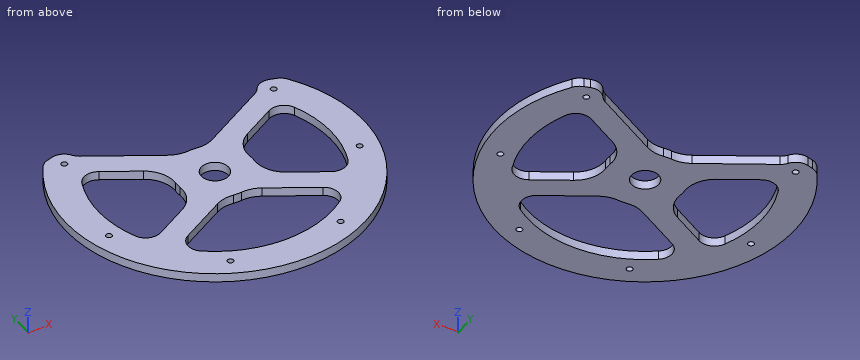
Autodesk Inventor part; units mm, degrees
ref_plane "YZ Plane" through (0, 0, 0) normal (1, 0, 0) x (0, 1, 0)
ref_plane "XZ Plane" through (0, 0, 0) normal (0, 1, 0) x (-1, 0, 0)
ref_plane "XY Plane" through (0, 0, 0) normal (0, 0, 1) x (1, 0, 0)
sketch "スケッチ1" plane through (0, 0, 0) normal (0, 0, 1) x (1, 0, 0)
  circle A0 centre (69, 50) radius 2
  circle A1 centre (0, 0) radius 9
  circle A2 centre (0, 0) radius 25
  circle A3 centre (69, 50) radius 7.5
  line L0 (65.25, 56.4952) -> (8.2643, 23.5945)
  line L1 (0, 25) -> (0, -25)
  line L2 (-25, 0) -> (25, 0)
  line L3 (20.9707, 13.61) -> (72.75, 43.5048)
  circle A4 centre (69, -50) radius 2
  circle A5 centre (69, -50) radius 7.5
  line L4 (65.25, -56.4952) -> (8.2643, -23.5945)
  line L5 (20.9707, -13.61) -> (72.75, -43.5048)
  circle A6 centre (-69, 50) radius 2
  circle A7 centre (-69, 50) radius 7.5
  line L6 (-65.25, 56.4952) -> (-8.2643, 23.5945)
  line L7 (-20.9707, 13.61) -> (-72.75, 43.5048)
  line L8 (-65.25, -56.4952) -> (-8.2643, -23.5945)
  circle A8 centre (-69, -50) radius 7.5
  circle A9 centre (-69, -50) radius 2
  line L9 (-20.9707, -13.61) -> (-72.75, -43.5048)
  circle A10 centre (0, 0) radius 77
  circle A11 centre (0, 0) radius 86.5
  circle A12 centre (0, 0) radius 98.5
  line L10 (0, 0) -> (79.6882, 57.8968)
  line L11 (0, 0) -> (95.4054, -24.496)
  line L12 (0, 0) -> (41.9393, -89.1255)
  line L13 (0, 0) -> (-79.6882, 57.8968)
  line L14 (0, 0) -> (-95.4054, -24.496)
  line L15 (0, 0) -> (-41.9393, -89.1255)
  circle A13 centre (69.98, 50.8434) radius 2
  circle A14 centre (83.7824, -21.5117) radius 2
  circle A15 centre (36.8299, -78.2675) radius 2
  circle A16 centre (69.98, 50.8434) radius 9.5
  circle A17 centre (-69.98, 50.8434) radius 2
  circle A18 centre (-83.7824, -21.5117) radius 2
  circle A19 centre (-36.8299, -78.2675) radius 2
  circle A20 centre (-69.98, 50.8434) radius 9.5
  line L16 (-79.6882, 57.8968) -> (-72.6529, 59.9596)
  line L17 (79.6882, 57.8968) -> (72.6529, 59.9596)
  point P0 (-8.2643, 23.5945)
  point P1 (-8.2643, -23.5945)
  point P2 (8.2643, -23.5945)
  point P3 (66.0238, -39.6214)
  point P4 (57.0218, -51.7447)
  point P5 (-57.0218, -51.7447)
  point P6 (-66.0238, -39.6214)
  point P7 (-66.0238, 39.6214)
  point P8 (-57.0218, 51.7447)
  point P9 (-62.2943, 45.2595)
  point P10 (-77.6656, 56.4274)
  point P11 (77.6656, 56.4274)
  point P12 (62.2943, 45.2595)
  point P13 (57.0218, 51.7447)
  point P14 (66.0238, 39.6214)
  point P15 (-61.0434, 54.0665)
  point P16 (61.0434, 54.0665)
  point P17 (69.0803, 41.3861)
  point P18 (-69.0803, 41.3861)
  point P19 (-12.1615, -25.8445)
  point P20 (-10.6445, -22.6207)
  point P21 (10.6445, -22.6207)
  point P22 (12.1615, -25.8445)
  dimension "d19" = 19
  dimension "d0" = 4
  dimension "d1" = 50
  dimension "d2" = 69
  dimension "d3" = 18
  dimension "d4" = 50
  dimension "d5" = 15
  dimension "d6" = 30
  dimension "d10" = 154
  dimension "d11" = 173
  dimension "d12" = 197
  dimension "d13" = 54
  dimension "d14" = 50.4
  dimension "d15" = 50.4
  dimension "d16" = 4
  dimension "d17" = 4
  dimension "d18" = 4
extrude "押し出し1" add sketch "スケッチ1" along normal blind 5.8 contours A13 A11 A3 L10 | L10 A3 A11 A13 | A13 A11 A3 L10 A0 | A0 L10 A13 | A13 L10 A0 | A0 L10 A3 A11 A13 | L10 A16 A11 A3 | A3 A11 A16 L10 | A11 A16 L3 A3 | A3 L0 A16 A11 | A16 L17 L10 | L10 A12 L11 A14 A11 A16 | L10 A16 L0 A3 | A3 L3 A16 L10 | A11 A14 L11 A10 L3 A16 | A16 L3 A10 | L10 A2 L0 A10 | A10 L3 A2 L10 | A10 L0 A16 | A20 L6 A7 A11 | A11 A7 L13 A20 | L13 A20 A11 A18 L14 A12 | L16 A20 L13 | L10 A1 L1 A2 | A2 L2 A1 L10 | A11 A17 L13 A7 | A7 L13 A6 A17 A11 | A20 L13 A7 L6 | L6 A10 A20 | A12 L12 A15 A11 A5 A14 L11 | L14 A18 A11 A8 A19 L15 A12 | L13 A7 A11 A20 | L6 A2 L13 A10 | A14 A11 A5 L5 A10 L11 | L13 A17 A11 A7 | A12 L15 A19 A11 A15 L12 | A20 L7 A10 L14 A18 A11 | A11 A7 L7 A20 | A2 L11 A1 L2 | L1 A1 L13 A2 | L13 A2 L7 A10 | A20 L7 A7 L13 | A10 L7 A20 | A11 A17 A6 L13 A7 | A6 L13 A17 | A18 L14 A10 L9 A8 A11 | A2 L12 A1 L11 | A10 L4 L12 A2 L5 | L5 A5 L4 A10 | L13 A1 L2 A2 | L1 A2 L15 A1 | A1 L12 A2 L1 | A1 L14 A2 L2 | A1 L15 A2 L14 | A11 A4 A5 | A5 A11 A4 | A11 A19 L15 A10 L12 A15 | A11 A8 L8 A10 L15 A19 | A11 A9 A8 | A8 A11 A9 | L4 A5 A11 A15 L12 A10 | A6 A17 L13 | L12 L4 A2 | L15 L8 A10 L9 A2 | A2 L8 L15 | A11 A4 | A4 A11 | L9 A10 L8 A8 | A11 A9 | A9 A11
fillet "フィレット1" radius 20 8 edges at (-8.2643, 23.5945, 2.9) (8.2643, 23.5945, 2.9) (-8.2643, -23.5945, 2.9) (8.2643, -23.5945, 2.9) (-20.9707, -13.61, 2.9) (-20.9707, 13.61, 2.9) (20.9707, 13.61, 2.9) (20.9707, -13.61, 2.9)
fillet "フィレット2" radius 10 10 edges at (-61.0434, 54.0665, 2.9) (61.0434, 54.0665, 2.9) (66.0238, 39.6214, 2.9) (66.0238, -39.6214, 2.9) (57.0218, -51.7447, 2.9) (-57.0218, -51.7447, 2.9) (-66.0238, -39.6214, 2.9) (-66.0238, 39.6214, 2.9) (79.6882, 57.8968, 2.9) (-79.6882, 57.8968, 2.9)
equation "\"d15\" = d14"
properties part number "TH22_POM_X" material "ABS プラスチック"
The listing builds one solid part. Answer for the finished solid, in the listing's coordinates (mm). Coordinates: 2 decimals unless noted, no trailing zeros. Order: outer loops, then holes, each group sorted by start corner. A loop starts at its lowest first (then second) coordinate and runs counter-clockwise, first axis right, second up. Notation, with made-up numbers: M 2,1.25 L 44,1.25 A24 cw 44,24.25 Z; hole C -29,37.5 d9. An arc over 180 degrees is marked long. Answer as a JSON object with one key per item and string values. Group by question number.
1. Section B-B on x = 0 is taken. Write down the section's boundary in (y, z).
2. Straight lines are drawn through the part: line 1 (Y direction, x = 0, z = 4.65); line 2 (X direction, y = 0, z = 3.5); line 3 (X direction, y = 19, z = 0.85). For each, find the intervals that lie inside material, in ascending order.
3. Section C-C on y = 19 is taken. Write down the section's boundary in (x, z), then the cut area to 3 significant figures.
4. Flat-ended cylindrical pins translate along their axes: P1, Ø6.5, axis at x = -69.98, y = 50.84, coming from the -Z side; P2, Ø2, axis at x = -9.5, z = 1, coming from the +Y side; P3, Ø2, axis at x = -50.5, z = 5, coming from the -Y side; P4, Ø2, axis at y = -82, z = 1.5, coming from the +X side. Find the tip coordinate at first contact, or state that the pin passes through.
5. Section A-A on y = 0 is taken. Write down the section's boundary in (x, z), then the cut area to 3 significant figures.
6. Section D-D on z = 4.55 is taken. State how many separate pieces and enclosed holes the cut face has, then the cut area to 3 significant figures.
Values follow:
{
 "1": {"outline": "M -98.5,0 L -77,0 L -77,5.8 L -98.5,5.8 Z; M -25,0 L -9,0 L -9,5.8 L -25,5.8 Z; M 9,0 L 25,0 L 25,5.8 L 9,5.8 Z"},
 "2": {"line 1": "-98.5 to -77, -25 to -9, 9 to 25", "line 2": "-98.5 to -77, -25 to -9, 9 to 25, 77 to 98.5", "line 3": "-96.65 to -74.62, -31.27 to 31.27, 74.62 to 96.65"},
 "3": {"outline": "M -96.65,0 L -74.62,0 L -74.62,5.8 L -96.65,5.8 Z; M -31.27,0 L 31.27,0 L 31.27,5.8 L -31.27,5.8 Z; M 74.62,0 L 96.65,0 L 96.65,5.8 L 74.62,5.8 Z", "area": "618 mm2"},
 "4": {"P1": "z = 0", "P2": "y = 25.54", "P3": "y = -85.16", "P4": "x = 56.05"},
 "5": {"outline": "M -98.5,0 L -77,0 L -77,5.8 L -98.5,5.8 Z; M -25,0 L -9,0 L -9,5.8 L -25,5.8 Z; M 9,0 L 25,0 L 25,5.8 L 9,5.8 Z; M 77,0 L 98.5,0 L 98.5,5.8 L 77,5.8 Z", "area": "435 mm2"},
 "6": {"separate pieces": "1", "enclosed holes": "10", "area": "13,800 mm2"}
}
